Source: CAD feature listing. Evaluate the final solid. Frame: model axes, mm. A direction names the side the tool comes from. Give positions to 0.01 mm unless a question says otherwise; leave off trailing zeros. Write each loop counter-clockwise with the first axis right and the second up, starting at its lowest first coordinate (ties: lowest second). Pieces come first, ordered by that corner, then holes. Notation, with made-up numbers: (86.5, -11.75) -> (94.5, -11.75) arc R25 ccw to (94.5, 15.25) -> close; hole circle Ø10 at (30.25, 86.5). An arc over 180 degrees is marked (long way). Write item = value, one per line.
from build123d import *

# Parameters (mm, degrees)
F0_W      = 250
F0_H      = 153
F1_DEPTH  = 260
F2_W      = 231
F2_H      = 190
F3_DEPTH  = 265
F4_W      = 150
F4_H      = 233
F5_DEPTH  = 190
F6_W      = 170
F6_H      = 240
F7_DEPTH  = 10
F8_W      = 151
F8_H      = 170
F9_DEPTH  = 15
F10_W     = 25
F10_H     = 7
F11_DEPTH = 40
F12_W     = 8
F12_H     = 7
F13_DEPTH = 13
F14_R     = 12
F15_DEPTH = 7
F16_R     = 10
F17_DEPTH = 7
F18_W     = 50.8
F18_H     = 25.4
F19_DEPTH = 9
F20_W     = 50.8
F20_H     = 25.4
F21_DEPTH = 9
F22_W     = 50.8
F22_H     = 25.4
F23_DEPTH = 9
F24_W     = 50.8
F24_H     = 25.4
F25_DEPTH = 9


with BuildPart() as f1:
    # F0 (on Front) → F1 (new body)
    with BuildSketch(Plane.XZ):
        Rectangle(F0_W, F0_H)
    extrude(amount=F1_DEPTH)

    # F2 (on face) → F3 (join)
    with BuildSketch(Plane.XY.offset(76.5)):
        with Locations((0, -128.47054)):
            Rectangle(F2_W, F2_H)
    extrude(amount=F3_DEPTH)

    # F4 (on face) → F5 (cut)
    with BuildSketch(Plane.XZ.offset(223.47054)):
        with Locations((30.5, 210)):
            Rectangle(F4_W, F4_H)
    extrude(amount=-F5_DEPTH, mode=Mode.SUBTRACT)

    # F6 (on face) → F7 (cut)
    with BuildSketch(Plane.YZ.offset(115.5)):
        with Locations((-128.47054, 213.5)):
            Rectangle(F6_W, F6_H)
    extrude(amount=-F7_DEPTH, mode=Mode.SUBTRACT)

    # F8 (on face) → F9 (cut)
    with BuildSketch(Plane.XY.offset(341.5)):
        with Locations((30, -128.47054)):
            Rectangle(F8_W, F8_H)
    extrude(amount=-F9_DEPTH, mode=Mode.SUBTRACT)

    # F10 (on face) → F11 (join)
    with BuildSketch(Plane.YZ.offset(-44.5)):
        with Locations((-128.371669, 211.050056)):
            Rectangle(F10_W, F10_H)
    extrude(amount=F11_DEPTH)

    # F12 (on face) → F13 (join)
    with BuildSketch(Plane.YZ.offset(-4.5)):
        with Locations((-128.627784, 211.050056)):
            Rectangle(F12_W, F12_H)
    extrude(amount=F13_DEPTH)

    # F14 (on face) → F15 (join)
    with BuildSketch(Plane.XY.offset(214.550056)):
        with Locations((20.38017, -130.319401)):
            Circle(F14_R)
    extrude(amount=-F15_DEPTH)

    # F16 (on face) → F17 (cut)
    with BuildSketch(Plane.XY.offset(214.550056)):
        with Locations((20.38017, -130.319401)):
            Circle(F16_R)
    extrude(amount=-F17_DEPTH, mode=Mode.SUBTRACT)

    # F18 (on face) → F19 (join)
    with BuildSketch(Plane(origin=(0, 0, -76.5), x_dir=(1, 0, 0), z_dir=(0, 0, -1))):
        with Locations((-74.2, 221.9)):
            Rectangle(F18_W, F18_H)
    extrude(amount=F19_DEPTH)

    # F20 (on face) → F21 (join)
    with BuildSketch(Plane(origin=(0, 0, -76.5), x_dir=(1, 0, 0), z_dir=(0, 0, -1))):
        with Locations((74.2, 221.9)):
            Rectangle(F20_W, F20_H)
    extrude(amount=F21_DEPTH)

    # F22 (on face) → F23 (join)
    with BuildSketch(Plane(origin=(0, 0, -76.5), x_dir=(1, 0, 0), z_dir=(0, 0, -1))):
        with Locations((74.2, 38.1)):
            Rectangle(F22_W, F22_H)
    extrude(amount=F23_DEPTH)

    # F24 (on face) → F25 (join)
    with BuildSketch(Plane(origin=(0, 0, -76.5), x_dir=(1, 0, 0), z_dir=(0, 0, -1))):
        with Locations((-74.2, 38.1)):
            Rectangle(F24_W, F24_H)
    extrude(amount=F25_DEPTH)


solid = f1.part
1) Access query for faces 5 (the flat face through (74, -25.4, -81)), 6 (the flat face through (-53, -223.471, 178)), 7 (the flat face through (-48.8, -38, -81)). Directions: +Z, -Z, +X, -X, +Y, -Y. A direction counts if a zero-diameter tool reaches every point of the face in a straight line with its end or side. Return the directions, or none.
Computed:
face_5 = -Z, +X, -X, +Y
face_6 = +Z, +X, -X, -Y
face_7 = -Z, +Y, -Y
2) Cut plane B-B (x = 57). Return the cut outline in (y, z), then the cut area to 3 significant figures.
Computed:
outline = (-260, -76.5) -> (-234.6, -76.5) -> (-234.6, -85.5) -> (-209.2, -85.5) -> (-209.2, -76.5) -> (-50.8, -76.5) -> (-50.8, -85.5) -> (-25.4, -85.5) -> (-25.4, -76.5) -> (0, -76.5) -> (0, 76.5) -> (-33.47, 76.5) -> (-33.47, 93.5) -> (-223.47, 93.5) -> (-223.47, 76.5) -> (-260, 76.5) -> close; (-223.47, 326.5) -> (-213.47, 326.5) -> (-213.47, 341.5) -> (-223.47, 341.5) -> close; (-43.47, 326.5) -> (-33.47, 326.5) -> (-33.47, 341.5) -> (-43.47, 341.5) -> close
area = 43,800 mm²
3) Cut plane C-C (y = -72). Return the cut outline in (x, z), then the cut area to 4 significant figures.
Computed:
outline = (-125, -76.5) -> (125, -76.5) -> (125, 76.5) -> (115.5, 76.5) -> (115.5, 93.5) -> (-44.5, 93.5) -> (-44.5, 326.5) -> (-45.5, 326.5) -> (-45.5, 341.5) -> (-115.5, 341.5) -> (-115.5, 76.5) -> (-125, 76.5) -> close; (105.5, 333.5) -> (115.5, 333.5) -> (115.5, 341.5) -> (105.5, 341.5) -> close
area = 59,850 mm²
4) Draft query along Y for faces 1 (the flat face through (-45.5, -130, 334)), 2 (the flat face through (-2, 0, 1)), 3 (the flat face through (107, -43.471, 272)), 4 (the flat face through (105.5, -39, 208)). Return one class per face: pulls with the +Y half, pulls with the -Y half, needs draft (parallel to the pull), parting line crosses it, or undercut.
Computed:
face_1 = undercut
face_2 = pulls with the +Y half
face_3 = undercut
face_4 = needs draft
5) Contact query for flat-ended pins moving along their axis: pin 1 (2.5 mm diameter, centred on y = -226.5, z = -82, fed in from +X); pin 2 (3 mm diameter, centred on x = 15, y = -220.5, fed in from -Z); pin 3 (2 mm diameter, centred on y = -137.5, z = 210, fed in from +X). Output: stop coordinate, or through.
Computed:
pin_1 = 99.6
pin_2 = -76.5
pin_3 = 30.67
6) Material intervals for L1, parallel to Y at x = 114, z = 281; L2, parallel to Z at x = 93.5, y = -197.5; L3, parallel to Y at x = -54.5, z = 130, sorted ascending.
Computed:
L1 = -223.47 to -213.47, -43.47 to -33.47
L2 = -76.5 to 93.5
L3 = -223.47 to -33.47
7) Cut plane A-A (z = 120.5). Return the cut outline in (x, y).
Computed:
outline = (-115.5, -223.47) -> (-44.5, -223.47) -> (-44.5, -33.47) -> (-115.5, -33.47) -> close; (105.5, -223.47) -> (115.5, -223.47) -> (115.5, -213.47) -> (105.5, -213.47) -> close; (105.5, -43.47) -> (115.5, -43.47) -> (115.5, -33.47) -> (105.5, -33.47) -> close
8) Cut plane D-D (x = 17). Return the cut outline in (y, z).
Computed:
outline = (-260, -76.5) -> (0, -76.5) -> (0, 76.5) -> (-33.47, 76.5) -> (-33.47, 93.5) -> (-223.47, 93.5) -> (-223.47, 76.5) -> (-260, 76.5) -> close; (-223.47, 326.5) -> (-213.47, 326.5) -> (-213.47, 341.5) -> (-223.47, 341.5) -> close; (-141.83, 207.55) -> (-139.73, 207.55) -> (-139.73, 214.55) -> (-141.83, 214.55) -> close; (-120.91, 207.55) -> (-118.81, 207.55) -> (-118.81, 214.55) -> (-120.91, 214.55) -> close; (-43.47, 326.5) -> (-33.47, 326.5) -> (-33.47, 341.5) -> (-43.47, 341.5) -> close
